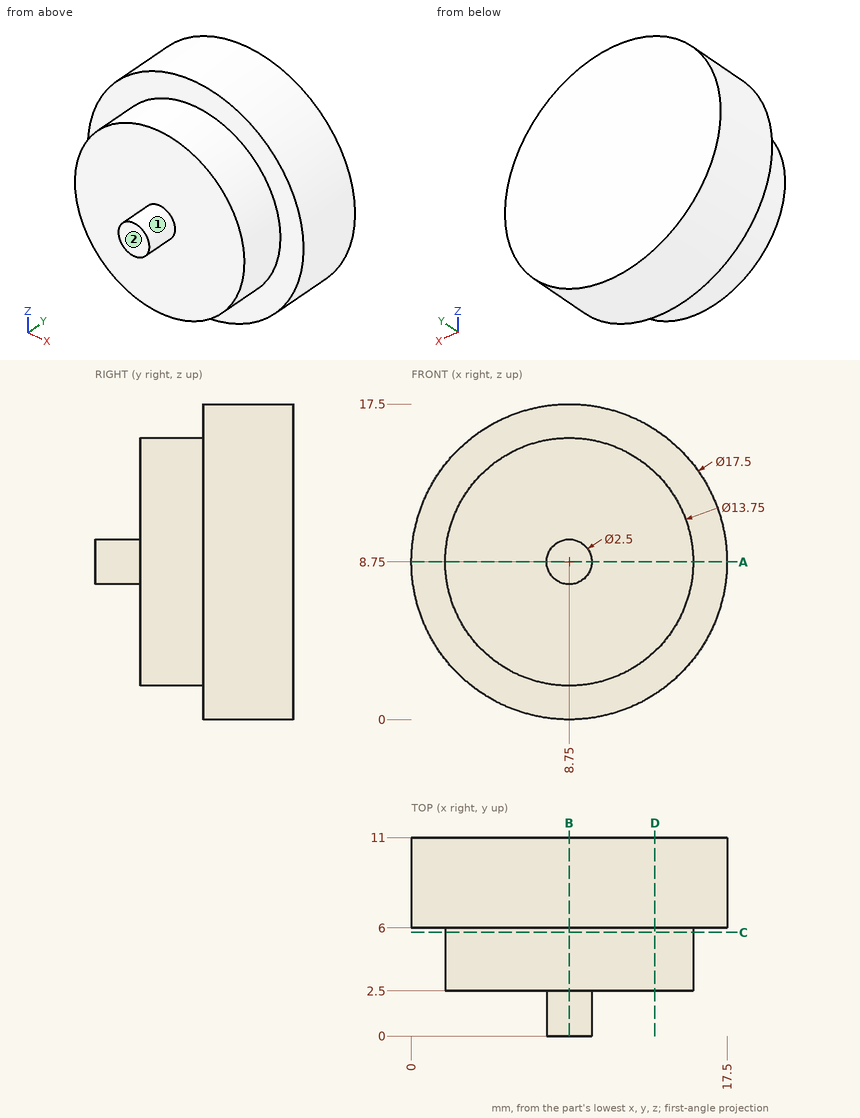
Geometry check sheet. Reference: drawing and pictorial views, mm from the part's lowest x, y, z. A direction names the side the tool comes from. Round coordinates to 2 decimals unless told otherwise and drop trailing zeros. Loops run counter-clockwise (first coordinate to the right, second up) from the corner with the lowest first, then second, coordinate; pieces in that order, holes last. Notation, with made-up numbers: (78.25, 81.5) -> (131.25, 81.5) arc R21 cw to (131.25, 116.5) -> close; hole circle Ø1 at (4, 49). An arc over 180 degrees is marked (long way). Answer as a JSON object with one key per item and string values. Group by question number.
Item 1: Depth check by flat-ended pin: pin 1 Ø2 at (x, z) = (14, 12) entering from -Y; pin 2 Ø3 at (y, z) = (7.5, 11) entering from +X; pin 3 Ø10 at (x, z) = (6, 4.5) entering from -Y; pin 4 Ø2 at (y, z) = (7.5, 14.5) entering from +X. Enter the tip coordinate at first touch or a pass-through.
Item 2: Cross-section at C-C, the plane y = 5.75. Record the cut outline in (x, z) (3 decimals), plus the area to 3 significant figures.
Item 3: Cross-section at A-A, the plane z = 8.75. Record the cut outline in (x, y) (3 decimals), plus the area to 3 significant figures.
Item 4: Set-up check for the marked faces 1 and 2: record each of +Z, -Z, +X, -X, +Y, -Y from which the full face is reachable in a straight line by a thin tool's end or side.
Item 5: Cross-section at D-D, the plane x = 13.5. Record the cut outline in (y, z), plus the area to 3 significant figures.
Item 6: Cross-section at B-B, the plane x = 8.75. Record the cut outline in (y, z) (3 decimals).
Item 7: Thickness scan on line 1 along Y through (x, z) = (5.25, 7); line 2 along Y through (x, z) = (13.25, 2); line 3 along Z through (x, y) = (8.5, 7). Record the ranges inside material, lowest first.
Determined:
{
 "1": {"pin 1": "stops at y = 2.5", "pin 2": "stops at x = 17.47", "pin 3": "stops at y = 0", "pin 4": "stops at x = 16.1"},
 "2": {"outline": "circle Ø13.75 at (8.75, 8.75)", "area": "148 mm²"},
 "3": {"outline": "(0, 6) -> (1.875, 6) -> (1.875, 2.5) -> (7.5, 2.5) -> (7.5, 0) -> (10, 0) -> (10, 2.5) -> (15.625, 2.5) -> (15.625, 6) -> (17.5, 6) -> (17.5, 11) -> (0, 11) -> close", "area": "142 mm²"},
 "4": {"face 1": "-Y", "face 2": "+Z, -Z, +X, -X, -Y"},
 "5": {"outline": "(2.5, 3.78) -> (6, 3.78) -> (6, 1.4) -> (11, 1.4) -> (11, 16.1) -> (6, 16.1) -> (6, 13.72) -> (2.5, 13.72) -> close", "area": "108 mm²"},
 "6": {"outline": "(0, 7.5) -> (2.5, 7.5) -> (2.5, 1.875) -> (6, 1.875) -> (6, 0) -> (11, 0) -> (11, 17.5) -> (6, 17.5) -> (6, 15.625) -> (2.5, 15.625) -> (2.5, 10) -> (0, 10) -> close"},
 "7": {"line 1": "y = 2.5 to 11", "line 2": "y = 6 to 11", "line 3": "z = 0 to 17.5"}
}
